from build123d import *

# Parameters (mm, degrees)
SKETCH1_R           = 1.5
BOSS_EXTRUDE2_DEPTH = 3
FILLET1_R           = 0.5
CUT_EXTRUDE1_DEPTH  = 3


with BuildPart() as part:
    # Sketch1 → Boss-Extrude2 (new body)
    with BuildSketch(Plane(origin=(0, 0, 0), x_dir=(1, 0, 0), z_dir=(0, 1, 0))):
        Polygon((15.5, -54), (34.5, -54), (50, -19), (50, 0), (0, 0), (0, -19), align=None)
        with Locations(Location((10, -9.5, 0), (0, 0, 270))):
            Circle(SKETCH1_R, mode=Mode.SUBTRACT)
        with Locations(Location((40, -9.5, 0), (0, 0, 270))):
            Circle(SKETCH1_R, mode=Mode.SUBTRACT)
        with Locations(Location((25, -44, 0), (0, 0, 270))):
            Circle(SKETCH1_R, mode=Mode.SUBTRACT)
        with Locations(Location((25, -29, 0), (0, 0, 270))):
            Circle(SKETCH1_R, mode=Mode.SUBTRACT)
        with Locations(Location((25, -9.5, 0), (0, 0, 270))):
            Circle(SKETCH1_R, mode=Mode.SUBTRACT)
    extrude(amount=BOSS_EXTRUDE2_DEPTH)

    # Fillet1
    fillet1_edges = [part.edges().sort_by_distance(p)[0] for p in [
        (50, 1.5, 0),
        (50, 1.5, 19),
        (34.5, 1.5, 54),
        (15.5, 1.5, 54),
        (0, 1.5, 19),
        (0, 1.5, 0),
    ]]
    fillet(fillet1_edges, radius=FILLET1_R)

    # Sketch2 → Cut-Extrude1 (cut)
    with BuildSketch(Plane(origin=(0, 3, 0), x_dir=(1, 0, 0), z_dir=(0, 1, 0))):
        with BuildLine():
            Line((6.189797727, -18.894239223), (18.120962557, -18.894239223))
            ThreePointArc((18.120962557, -18.894239223), (18.555574645, -19.147030136), (18.550722787, -19.649789891))
            Line((18.550722787, -19.649789891), (11.712415101, -31.149789891))
            ThreePointArc((11.712415101, -31.149789891), (11.25278078, -31.393345964), (10.825480175, -31.096702302))
            Line((10.825480175, -31.096702302), (5.732623032, -19.596702302))
            ThreePointArc((5.732623032, -19.596702302), (5.770732375, -19.121504498), (6.189797727, -18.894239223))
        make_face()
        with BuildLine():
            Line((18.070239769, -28.284056063), (13.335984482, -36.245665617))
            ThreePointArc((13.335984482, -36.245665617), (13.266637971, -36.471342196), (13.308570017, -36.703679365))
            Line((13.308570017, -36.703679365), (18.042825305, -47.39393324))
            ThreePointArc((18.042825305, -47.39393324), (18.603471379, -47.680646687), (19, -47.191470161))
            Line((19, -47.191470161), (19, -28.539606732))
            ThreePointArc((19, -28.539606732), (18.632513933, -28.057486355), (18.070239769, -28.284056063))
        make_face()
        with BuildLine():
            Line((38.287584899, -31.149789891), (31.449277213, -19.649789891))
            ThreePointArc((31.449277213, -19.649789891), (31.444425355, -19.147030136), (31.879037443, -18.894239223))
            Line((31.879037443, -18.894239223), (43.810202273, -18.894239223))
            ThreePointArc((43.810202273, -18.894239223), (44.229267625, -19.121504498), (44.267376968, -19.596702302))
            Line((44.267376968, -19.596702302), (39.174519825, -31.096702302))
            ThreePointArc((39.174519825, -31.096702302), (38.74721922, -31.393345964), (38.287584899, -31.149789891))
        make_face()
        with BuildLine():
            Line((31, -47.191470161), (31, -28.539606732))
            ThreePointArc((31, -28.539606732), (31.367486067, -28.057486355), (31.929760231, -28.284056063))
            Line((31.929760231, -28.284056063), (36.664015518, -36.245665617))
            ThreePointArc((36.664015518, -36.245665617), (36.733362029, -36.471342196), (36.691429983, -36.703679365))
            Line((36.691429983, -36.703679365), (31.957174695, -47.39393324))
            ThreePointArc((31.957174695, -47.39393324), (31.396528621, -47.680646687), (31, -47.191470161))
        make_face()
    extrude(amount=-CUT_EXTRUDE1_DEPTH, mode=Mode.SUBTRACT)


solid = part.part
Design review of the part built by this model. Coordinates are the model's own, in mm. A direction names the side the tool comes from. Coordinates: 2 decimals unless noted, no trailing zeros. Write each loop counter-clockwise with the first axis right and the second up, starting at its lowest first coordinate (ties: lowest second). Pieces come first, ordered by that corner, then holes. Notation, with made-up numbers: (-9, 12) - (0, 12) arc R19 ccw to (0, 24) - close; hole circle Ø6 at (33.5, 39.5). An arc over 180 degrees is marked (long way). One line per item, written item: value.
1) Add section C-C (z = 38). State the section outline as (x, y) points.
Answer sheet:
outline: (8.41, 0) - (13.88, 0) - (13.88, 3) - (8.41, 3) - close; (19, 0) - (31, 0) - (31, 3) - (19, 3) - close; (36.12, 0) - (41.59, 0) - (41.59, 3) - (36.12, 3) - close
2) Add section A-A (z = 9.5). State the section outline as (x, y) points.
Answer sheet:
outline: (0, 0) - (8.5, 0) - (8.5, 3) - (0, 3) - close; (11.5, 0) - (23.5, 0) - (23.5, 3) - (11.5, 3) - close; (26.5, 0) - (38.5, 0) - (38.5, 3) - (26.5, 3) - close; (41.5, 0) - (50, 0) - (50, 3) - (41.5, 3) - close
3) Insertion check: pin 1 (1.5 mm diameter, centred on x = 37, y = 2, fed in from +Z); pin 2 (0.9 mm diameter, centred on y = 1.5, z = 36.5, fed in from -X); pin 3 (1.5 mm diameter, centred on y = 1, z = 42.5, fed in from +X) (3 decimals). Each pin has a flat end and moves straight along its axis. Give the tip position at first contact, or say it passes through.
Answer sheet:
pin 1: stops at z = 50.05
pin 2: stops at x = 7.55
pin 3: stops at x = 39.925
4) To check wall thickness, follow probe 1 along X at (y, z) = (1.5, 9.5); probe 2 along Z at (x, y) = (11, 1.3); probe 3 along X at (y, z) = (2.75, 35.5). State the ranges of each line that lie inside material, in increasing order.
Answer sheet:
probe 1: x = 0 to 8.5, 11.5 to 23.5, 26.5 to 38.5, 41.5 to 50
probe 2: z = 0 to 8.38, 10.62 to 18.89, 31.31 to 43.84
probe 3: x = 7.31 to 13.78, 19 to 31, 36.22 to 42.69
5) Add section D-D (z = 44). State the section outline as (x, y) points.
Answer sheet:
outline: (11.07, 0) - (16.54, 0) - (16.54, 3) - (11.07, 3) - close; (19, 0) - (23.5, 0) - (23.5, 3) - (19, 3) - close; (26.5, 0) - (31, 0) - (31, 3) - (26.5, 3) - close; (33.46, 0) - (38.93, 0) - (38.93, 3) - (33.46, 3) - close
6) Add section B-B (x = 10). State the section outline as (y, z) points.
Answer sheet:
outline: (0, 0) - (3, 0) - (3, 8) - (0, 8) - close; (0, 11) - (3, 11) - (3, 18.89) - (0, 18.89) - close; (0, 29.23) - (3, 29.23) - (3, 41.58) - (0, 41.58) - close
7) Mouldability with a two-part tool opening along X and no side actions: class faces 1 (the face through (25, 1, 54)), 2 (the face through (34.264, 1.521, 32.209)) as +X half, -X half, draft (parallel to the pull), parting line (faces both ways), or undercut.
Answer sheet:
face 1: draft
face 2: undercut
8) For faces 3 (the face through (8.315, 1.521, 25.427)), 4 (the face through (25, 0, 21)), list the 3-axis set-ups (+Z, -Z, +X, -X, +Y, -Y) from which the entire face can be reached by the end or side of a thin tool; tool diameter is ignored.
Answer sheet:
face 3: +Y, -Y
face 4: +Z, -Z, +X, -X, -Y
